The listing builds one solid part. Answer for the finished solid, in the listing's coordinates (mm). A direction names the side the tool comes from. Coordinates: 2 decimals unless noted, no trailing zeros. Write each loop counter-clockwise with the first axis right and the second up, starting at its lowest first coordinate (ties: lowest second). Pieces come first, ordered by that corner, then holes. Notation, with made-up numbers: M 88,27.25 L 127,27.25 A22 cw 127,37.25 Z; hole C -10,-22.75 d1. An arc over 180 degrees is marked long. Answer as CSV lines item,"result".
Autodesk Inventor part; units mm, degrees
ref_plane "YZ Plane" through (0, 0, 0) normal (1, 0, 0) x (0, 1, 0)
ref_plane "XZ Plane" through (0, 0, 0) normal (0, 1, 0) x (-1, 0, 0)
ref_plane "XY Plane" through (0, 0, 0) normal (0, 0, 1) x (1, 0, 0)
sketch "Sketch1" plane through (0, 0, 0) normal (0, 0, 1) x (1, 0, 0)
  line L0 (-17.386, 3.6293) -> (12.614, 3.6293)
  line L1 (12.614, 3.6293) -> (12.614, -9.6107)
  line L2 (12.614, -9.6107) -> (-17.386, -9.6107)
  line L3 (-17.386, -9.6107) -> (-17.386, 3.6293)
  point P0 (0, 0)
  dimension "d0" = 30
  dimension "d1" = 13.24
extrude "Extrusion1" add sketch "Sketch1" along normal blind 5
sketch "Sketch2" plane through (0, 0, 5) normal (0, 0, 1) x (1, 0, 0)
  line L0 (12.614, 3.6293) -> (-17.386, 3.6293)
  line L1 (-17.386, 3.6293) -> (-17.386, -9.6107)
  line L2 (12.614, 3.6293) -> (-17.386, 3.6293)
  line L3 (-17.386, 3.6293) -> (-17.386, -1.3707)
  line L4 (-17.386, -1.3707) -> (12.614, -1.3707)
  line L5 (12.614, -1.3707) -> (12.614, 3.6293)
  line L6 (12.614, -9.6107) -> (12.614, 3.6293)
  line L7 (-17.386, -9.6107) -> (12.614, -9.6107)
  line L8 (12.614, -9.6107) -> (12.614, -4.6107)
  line L9 (12.614, -4.6107) -> (-17.386, -4.6107)
  line L10 (-17.386, -4.6107) -> (-17.386, -9.6107)
  point P0 (0, 0)
  dimension "d4" = 5
  dimension "d5" = 5
extrude "Extrusion2" add sketch "Sketch2" along normal blind 2 contours L5 L4 L1 L0 | L6 L7 L1 L9
sketch "Sketch3" plane through (0, 0, 7) normal (0, 0, 1) x (1, 0, 0)
  line L0 (-2.386, 3.6293) -> (-2.386, -9.6107) construction
  line L1 (2.714, 3.6293) -> (-7.486, 3.6293)
  line L2 (-7.486, 3.6293) -> (-7.486, -1.3707)
  line L3 (-7.486, -1.3707) -> (2.714, -1.3707)
  line L4 (2.714, -1.3707) -> (2.714, 3.6293)
  line L5 (12.614, -2.9907) -> (-17.386, -2.9907) construction
  line L6 (2.714, -9.6107) -> (-7.486, -9.6107)
  line L7 (-7.486, -9.6107) -> (-7.486, -4.6107)
  line L8 (-7.486, -4.6107) -> (2.714, -4.6107)
  line L9 (2.714, -4.6107) -> (2.714, -9.6107)
  point P0 (0, 0)
  point P1 (12.614, -9.6107)
  point P2 (-17.386, -9.6107)
  dimension "d8" = 10.2
extrude "Extrusion3" add sketch "Sketch3" along normal blind 6
sketch "Sketch4" plane through (0, 0, 13) normal (0, 0, 1) x (1, 0, 0)
  line L0 (2.714, 3.6293) -> (-7.486, 3.6293)
  line L1 (-2.386, 3.6293) -> (-2.386, -9.6107) construction
  line L2 (-7.486, -9.6107) -> (2.714, -9.6107)
  line L3 (-2.286, 3.6293) -> (-2.486, 3.6293)
  line L4 (-2.486, 3.6293) -> (-2.486, -9.6107)
  line L5 (-2.486, -9.6107) -> (-2.286, -9.6107)
  line L6 (-2.286, -9.6107) -> (-2.286, 3.6293)
  point P0 (0, 0)
  dimension "d11" = 0.2
extrude "Extrusion4" cut sketch "Sketch4" against normal blind 10
properties part number "BalsaBoi"
Q1. Find section B-B (x = -12.75). Give the vertices of the cut face in (y, z).
Output:
outline,"M -9.61,0 L 3.63,0 L 3.63,7 L -1.37,7 L -1.37,5 L -4.61,5 L -4.61,7 L -9.61,7 Z"
Q2. Flat-ended cylindrical pins translate along their axes: pin 1 Ø1.5 at (y, z) = (1.5, 11) entering from +X; pin 2 Ø4 at (x, z) = (3.5, 9) entering from +Y; pin 3 Ø1.5 at (y, z) = (2, 9.5) entering from -X; pin 4 Ø1.6 at (x, y) = (-10.5, -3.5) entering from +Z. Find the tip coordinate at first contact, or state that the pin passes through.
Output:
pin 1,"x = 2.71"
pin 2,"y = 3.63"
pin 3,"x = -7.49"
pin 4,"z = 5"
Q3. Find section C-C (y = -3). Give the vertices of the cut face in (x, z), and give its area (3 significant figures).
Output:
outline,"M -17.39,0 L 12.61,0 L 12.61,5 L -2.29,5 L -2.29,3 L -2.49,3 L -2.49,5 L -17.39,5 Z"
area,"150 mm2"
Q4. For faces 4 (the flat face through (2.714, -7, 10)), 5 (the flat face through (-13, 1, 7)), 6 (the flat face through (5, -3, 5)), determine the directions among +Z, -Z, +X, -X, +Y, -Y from which every point of the face is accessible in a straight line to the end or side of a thin tool.
Output:
face 4,"+Z, +X, +Y, -Y"
face 5,"+Z, -X, +Y, -Y"
face 6,"+Z, +X, -X"
Q5. Straight lines are drawn through the part: line 1 (X direction, y = -8.25, z = 11); line 2 (X direction, y = -7.25, z = 4.5); line 3 (Y direction, x = -16, z = 5.5). For each, find the intervals that lie inside material, in ascending order.
Output:
line 1,"-7.49 to -2.49, -2.29 to 2.71"
line 2,"-17.39 to -2.49, -2.29 to 12.61"
line 3,"-9.61 to -4.61, -1.37 to 3.63"
Q6. Find section D-D (z = 9). Give the vertices of the cut face in (x, y), and give its area (3 significant figures).
Output:
outline,"M -7.49,-9.61 L -2.49,-9.61 L -2.49,-4.61 L -7.49,-4.61 Z; M -7.49,-1.37 L -2.49,-1.37 L -2.49,3.63 L -7.49,3.63 Z; M -2.29,-9.61 L 2.71,-9.61 L 2.71,-4.61 L -2.29,-4.61 Z; M -2.29,-1.37 L 2.71,-1.37 L 2.71,3.63 L -2.29,3.63 Z"
area,"100 mm2"
Q7. Find section A-A (z = 5.5). Give the vertices of the cut face in (x, y), and give its area (3 significant figures).
Output:
outline,"M -17.39,-9.61 L -2.49,-9.61 L -2.49,-4.61 L -17.39,-4.61 Z; M -17.39,-1.37 L -2.49,-1.37 L -2.49,3.63 L -17.39,3.63 Z; M -2.29,-9.61 L 12.61,-9.61 L 12.61,-4.61 L -2.29,-4.61 Z; M -2.29,-1.37 L 12.61,-1.37 L 12.61,3.63 L -2.29,3.63 Z"
area,"298 mm2"
Q8. The mould has two halves that part along Y. Classify faces 1 (the flat face through (2.714, 1, 10)), 2 (the flat face through (-2, -9.611, 5)), 3 (the flat face through (-10, -3, 5)): pulls with the +Y half, pulls with the -Y half, needs draft (parallel to the pull), parting line crosses it, or undercut.
Output:
face 1,"needs draft"
face 2,"pulls with the -Y half"
face 3,"undercut"
